```python
from build123d import *

# Parameters (mm, degrees)
F1_DEPTH = 19
F2_R     = 2.5
F3_DEPTH = 48.001
F4_START = 8
F2_R_2   = 4.5
F4_DEPTH = 40.001
F5_R     = 5
F6_R     = 5


with BuildPart() as f1:
    # F0 (on Front) → F1 (new body)
    with BuildSketch(Plane.XZ):
        with BuildLine():
            Line((-70, 8), (-70, 0))
            Line((-70, 0), (70, 0))
            Line((70, 0), (70, 8))
            Line((70, 8), (65, 8))
            ThreePointArc((65, 8), (57.9289321881, 10.9289321881), (55, 18))
            Line((55, 18), (55, 28))
            ThreePointArc((55, 28), (49.1421356237, 42.1421356237), (35, 48))
            Line((35, 48), (-35, 48))
            ThreePointArc((-35, 48), (-49.1421356237, 42.1421356237), (-55, 28))
            Line((-55, 28), (-55, 18))
            ThreePointArc((-55, 18), (-57.9289321881, 10.9289321881), (-65, 8))
            Line((-65, 8), (-70, 8))
        make_face()
        with BuildLine():
            ThreePointArc((47.0360852778, 26.9401988387), (44.1071530897, 19.8691310268), (37.0360852778, 16.9401988387))
            Line((37.0360852778, 16.9401988387), (-37.0360852778, 16.9401988387))
            ThreePointArc((-37.0360852778, 16.9401988387), (-44.1071530897, 19.8691310268), (-47.0360852778, 26.9401988387))
            Line((-47.0360852778, 26.9401988387), (-47.0360852778, 29.0598011613))
            ThreePointArc((-47.0360852778, 29.0598011613), (-44.1071530897, 36.1308689732), (-37.0360852778, 39.0598011613))
            Line((-37.0360852778, 39.0598011613), (37.0360852778, 39.0598011613))
            ThreePointArc((37.0360852778, 39.0598011613), (44.1071530897, 36.1308689732), (47.0360852778, 29.0598011613))
            Line((47.0360852778, 29.0598011613), (47.0360852778, 26.9401988387))
        make_face(mode=Mode.SUBTRACT)
    extrude(amount=F1_DEPTH)

    # F2 (on Top) → F3 (cut, through all)
    with BuildSketch(Plane.XY):
        with Locations((-62.5, -9.5)):
            Circle(F2_R)
        with Locations((62.5, -9.5)):
            Circle(F2_R)
    extrude(amount=F3_DEPTH, mode=Mode.SUBTRACT)

    # F2 (on Top) → F4 (cut)
    with BuildSketch(Plane.XY.offset(F4_START)):
        with Locations((-62.5, -9.5)):
            Circle(F2_R_2)
        with Locations((-62.5, -9.5)):
            Circle(F2_R, mode=Mode.SUBTRACT)
        with Locations((62.5, -9.5)):
            Circle(F2_R_2)
        with Locations((62.5, -9.5)):
            Circle(F2_R, mode=Mode.SUBTRACT)
    extrude(amount=F4_DEPTH, mode=Mode.SUBTRACT)

    # F5
    f5_edges = [f1.edges().sort_by_distance(p)[0] for p in [
        (0, -19, 16.940199),
        (0, 0, 16.940199),
    ]]
    fillet(f5_edges, radius=F5_R)

    # F6
    f6_edges = [f1.edges().sort_by_distance(p)[0] for p in [
        (70, -19, 4),
        (70, 0, 4),
        (-70, -19, 4),
        (-70, 0, 4),
    ]]
    fillet(f6_edges, radius=F6_R)


solid = f1.part
```
The listing builds one solid part. Answer for the finished solid, in the listing's coordinates (mm). A direction names the side the tool comes from. Coordinates: 2 decimals unless noted, no trailing zeros. Write each loop counter-clockwise with the first axis right and the second up, starting at its lowest first coordinate (ties: lowest second). Pieces come first, ordered by that corner, then holes. Notation, with made-up numbers: (-25.75, 61) - (-18.75, 61) arc R13 cw to (-18.75, 76) - close; hole circle Ø8 at (-39.75, 56). An arc over 180 degrees is marked (long way). Return JSON: item names as keys, results as strings. Group by question number.
Q1. The part is cut by section A-A on y = -9.5. State how many separate pieces and enclosed holes the cut face has, and give its area (3 significant figures).
Q2. Which of the six approach directions +Z, -Z, +X, -X, +Y, -Y give full straight-line access (tool end or side, diameter ignored) to faces 1 (the cylindrical face through (0.52, -17.57, 40.56)), 2 (the flat face through (-1, -9, 39.06)), 3 (the cylindrical face through (-0.52, -1.5, 15.51)), 4 (the flat face through (70, -9, 4))?
Q3. The part is cut by section B-B on x = 12.5. Write down the section's boundary in (y, z), and give its area (3 significant figures).
Q4. For a pull along Z with two mould halves and no side action, classify faces 5 (the flat face through (0, 0, 8)), 6 (the flat face through (-65.2, -9.4, 8)), 7 (the flat face through (1, -9, 16.94)), 8 (the cylindrical face through (-48.462, -1.504, 28.015)) as +Z half, -Z half, draft (parallel to the pull), parting line (faces both ways), or undercut.
Q5. Flat-ended cylindrical pins translate along their axes: pin 1 Ø6 at (x, y) = (65.5, -8.5) entering from +Z; pin 2 Ø3 at (y, z) = (-9.5, 22.5) entering from +X; pin 3 Ø0.6 at (y, z) = (-10.5, 28.5) entering from -X. Find the tip coordinate at first contact, or state that the pin passes through.
Q6. Find the intervals of material crossed by line 1 along Z through (x, y) = (27, -11); line 2 along Y through (x, z) = (-62.5, 5.75); line 3 along X through (y, z) = (-1.5, 36.5), in increasing order. Write a range as [from, to].
Q7. The part is cut by section C-C on x = 62.5. Write down the section's boundary in (y, z).
Evaluation:
{
 "1": {"separate pieces": "3", "enclosed holes": "1", "area": "3,300 mm2"},
 "2": {"face 1": "-Y", "face 2": "+Y, -Y", "face 3": "+Y", "face 4": "+Z, -Z, +X, +Y, -Y"},
 "3": {"outline": "(-19, 0) - (0, 0) - (0, 11.94) arc R5 ccw to (-5, 16.94) - (-14, 16.94) arc R5 ccw to (-19, 11.94) - close; (-19, 44.06) arc R5 ccw to (-14, 39.06) - (-5, 39.06) arc R5 ccw to (0, 44.06) - (0, 48) - (-19, 48) - close", "area": "470 mm2"},
 "4": {"face 5": "draft", "face 6": "+Z half", "face 7": "undercut", "face 8": "undercut"},
 "5": {"pin 1": "stops at z = 8", "pin 2": "stops at x = 55", "pin 3": "stops at x = -55"},
 "6": {"line 1": "z = [0, 16.94], [39.06, 48]", "line 2": "y = [-19, -12], [-7, 0]", "line 3": "x = [-53.1, -45.71], [45.71, 53.1]"},
 "7": {"outline": "(-19, 0) - (-12, 0) - (-12, 8) - (-14, 8) - (-14, 8.32) - (-19, 8.32) - close; (-7, 0) - (0, 0) - (0, 8.32) - (-5, 8.32) - (-5, 8) - (-7, 8) - close"}
}
